Autodesk Inventor part; units mm, degrees
ref_plane "Start Plane" through (0, 0, 80) normal (0, 0, 1) x (1, 0, 0)
ref_plane "End Plane" through (0, 0, 234.949) normal (0, 0, 1) x (1, 0, 0)
ref_plane "Work Plane4" through (14, 23.6837, 221.6816) normal (0, 0.204, 0.979) x (1, 0, 0)
ref_plane "Start Plane" through (0, 0, 80) normal (0, 0, 1) x (1, 0, 0)
ref_plane "End Plane" through (0, 0, 234.949) normal (0, 0, 1) x (1, 0, 0)
sketch "Sketch" plane through (0, 0, 0) normal (0, 0, 1) x (1, 0, 0)
  line L0 (-20, -34) -> (-20, 34)
  line L1 (-14, 40) -> (14, 40)
  line L2 (20, 34) -> (20, -34)
  line L3 (14, -40) -> (-14, -40)
  arc A0 (-20, -34) -> (-14, -40) centre (-14, -34) ccw
  arc A1 (20, 34) -> (14, 40) centre (14, 34) ccw
  arc A2 (-14, 40) -> (-20, 34) centre (-14, 34) ccw
  arc A3 (14, -40) -> (20, -34) centre (14, -34) ccw
  arc A4 (-14, 37) -> (-17, 34) centre (-14, 34) ccw
  line L4 (-14, 37) -> (14, 37)
  arc A5 (17, 34) -> (14, 37) centre (14, 34) ccw
  line L5 (17, 34) -> (17, -34)
  arc A6 (14, -37) -> (17, -34) centre (14, -34) ccw
  line L6 (14, -37) -> (-14, -37)
  arc A7 (-17, -34) -> (-14, -37) centre (-14, -34) ccw
  line L7 (-17, -34) -> (-17, 34)
  line L8 (0, 57.7397) -> (0, -57.7397) construction
  line L9 (-29.7397, 0) -> (29.7397, 0) construction
  dimension "d7" = 6
  dimension "d9" = 40
  dimension "d11" = 80
  dimension "d12" = 3
  dimension "d15" = 20
  dimension "d16" = 40
extrude "Body" add sketch "Sketch" along normal up to surface (154.949 mm away) from surface at 80
sketch "Sketch3" plane through (0, 0, 0) normal (0, 0, 1) x (1, 0, 0)
  line L0 (0, 0) -> (10, 0)
ref_plane "Work Plane3" through (0, 0, 0) normal (0, -1, 0) x (1, 0, 0)
ref_plane "Work Plane4" through (14, 23.6837, 221.6816) normal (0, 0.204, 0.979) x (1, 0, 0)
split "Split1" plane through (14, 23.6837, 221.6816) removes the side toward (0, 0.204, 0.979)
sketch "Sketch4" plane through (0, 0, 0) normal (0, -1, 0) x (1, 0, 0)
  line L0 (-2, 80) -> (12, 80)
  line L1 (-2, 234.949) -> (12, 234.949)
  dimension "d18" = 154.949
equation "\"d7\" = G_IR"
equation "\"d9\" = G_W"
equation "\"d11\" = G_H"
equation "\"d12\" = G_T"
equation "\"d15\" = 0.5 * d9"
equation "\"d16\" = 0.5 * d11"
equation "\"d3\" = G_L"
equation "\"G_W\" = 40"
equation "\"G_H\" = 80"
equation "\"G_T\" = 3"
equation "\"G_IR\" = 6"
equation "\"G_L\" = d18"
equation "\"G_OFFSET_END\" = -65.051"
equation "\"d14\" = G_OFFSET_END + B_L"
properties part number "ISO 10799-2 - 80x40x3 - 154.95" material "Steel, Mild"
Design review of the part built by this model. Coordinates are the model's own, in mm. A direction names the side the tool comes from. Coordinates: 2 decimals unless noted, no trailing zeros. Write each loop counter-clockwise with the first axis right and the second up, starting at its lowest first coordinate (ties: lowest second). Pieces come first, ordered by that corner, then holes. Notation, with made-up numbers: (6.5, 46.25) -> (18.5, 46.25) arc R16 ccw to (18.5, 69.25) -> close; hole circle Ø9 at (71.25, -17). An arc over 180 degrees is marked (long way). Write each question's results on one line, items separated by ' | '. Start each with the question number.
(1) Tool access review of faces 1 (the face through (0, 37, 148)), 2 (the face through (20, 0, 156)): name each direction out of +Z, -Z, +X, -X, +Y, -Y from which nothing blocks a thin tool from reaching the whole face with its end or side.
(2) Take a section at B-B on z = 177. Write out the cut boundary in (x, y), and give its area (3 significant figures).
(3) Clearance check with a flat-ended pin moving along its axis: P1, Ø1.5, axis at x = 15, y = 20.5, coming from the +Z side. State where the tip first meets the part, or that it passes through.
(4) For line 1 along Y through (x, z) = (3.5, 203); line 2 along X through (y, z) = (-20, 173); line 3 along Y through (x, z) = (-13.5, 223.5), list the stretches that pass through material, from the lowest coordinate up. Write a range as from..to.
(5) Take a section at C-C on y = 4.5. Write out the cut boundary in (x, z).
(6) The part is to be moulded in two halves that separate along Y. For faces 3 (the face through (-18.289, 38.196, 148.789)), 4 (the face through (0, -37, 156)), 5 (the face through (18.289, -38.196, 156.39)), say which applies: pulls with the +Y half, pulls with the -Y half, needs draft (parallel to the pull), parting line crosses it, or undercut.
(7) Take a section at D-D on y = -31. Write out the cut boundary in (x, z), and give its area (3 significant figures).
Results found:
1) face 1: +Z, -Z | face 2: +Z, -Z, +X, +Y, -Y
2) outline: (-20, -34) arc R6 ccw to (-14, -40) -> (14, -40) arc R6 ccw to (20, -34) -> (20, 34) arc R6 ccw to (14, 40) -> (-14, 40) arc R6 ccw to (-20, 34) -> close; hole (-17, -34) arc R3 ccw to (-14, -37) -> (14, -37) arc R3 ccw to (17, -34) -> (17, 34) arc R3 ccw to (14, 37) -> (-14, 37) arc R3 ccw to (-17, 34) -> close | area: 661 mm2
3) P1: passes through
4) line 1: y = -40..-37, 37..40 | line 2: x = -20..-17, 17..20 | line 3: y = -40..-37
5) outline: (-20, 80) -> (-17, 80) -> (-17, 225.68) -> (-20, 225.68) -> close; (17, 80) -> (20, 80) -> (20, 225.68) -> (17, 225.68) -> close
6) face 3: pulls with the +Y half | face 4: undercut | face 5: pulls with the -Y half
7) outline: (-20, 80) -> (-17, 80) -> (-17, 233.08) -> (-20, 233.08) -> close; (17, 80) -> (20, 80) -> (20, 233.08) -> (17, 233.08) -> close | area: 918 mm2
